```python
from build123d import *

# Parameters (mm, degrees)
SALIENTE_EXTRUIR1_DEPTH = 170
CROQUIS2_W              = 271.012090605
CROQUIS2_H              = 220
SALIENTE_EXTRUIR2_DEPTH = 2


with BuildPart() as part:
    # Croquis1 → Saliente-Extruir1 (new body)
    with BuildSketch(Plane(origin=(0, 0, 0), x_dir=(1, 0, 0), z_dir=(0, 1, 0))):
        Polygon((-305.737821636, -89.613714521), (-305.737821636, 100.579273879), (350.262178364, 100.579273879), (350.262178364, -117.420726121), (352.262178364, -117.420726121), (352.262178364, 102.579273879), (-307.737821636, 102.579273879), (-307.737821636, -89.613714521), align=None)
    extrude(amount=SALIENTE_EXTRUIR1_DEPTH)

    # Croquis2 → Saliente-Extruir2 (add)
    with BuildSketch(Plane(origin=(0, 170, 0), x_dir=(1, 0, 0), z_dir=(0, 1, 0))):
        with Locations((-172.231776334, -7.420726121)):
            Rectangle(CROQUIS2_W, CROQUIS2_H)
    extrude(amount=SALIENTE_EXTRUIR2_DEPTH)


solid = part.part
```
Here's how the part is built. I have some questions about the finished solid (model axes, mm). A direction names the side the tool comes from. Coordinates: 2 decimals unless noted, no trailing zeros. Loops run counter-clockwise (first coordinate to the right, second up) from the corner with the lowest first, then second, coordinate; pieces in that order, holes last. Notation, with made-up numbers: (15, 39) - (71, 39) arc R25 ccw to (71, 53) - close; hole circle Ø10 at (6, 12). An arc over 180 degrees is marked (long way). Answer as CSV lines item,"result".
Q1. If we section it at C-C, the plane x = -56: Write out the boundary of the cut face in (y, z), and give its area (3 significant figures).
Response:
outline,"(0, -102.58) - (172, -102.58) - (172, 117.42) - (170, 117.42) - (170, -100.58) - (0, -100.58) - close"
area,"780 mm2"
Q2. For faces 5 (the face through (350.262, 84, 7)), 6 (the face through (18, 85, -102.579)), 7 (the face through (18, 84, -100.579)), which set-ups out of +Z, -Z, +X, -X, +Y, -Y let a thin tool reach every point of the face, with its end or its side?
Response:
face 5,"+Z, +Y, -Y"
face 6,"-Z, +X, -X, +Y, -Y"
face 7,"+Z, -Y"
Q3. If we section it at D-D, the plane x = 278: Write out the boundary of the cut face in (y, z).
Response:
outline,"(0, -102.58) - (170, -102.58) - (170, -100.58) - (0, -100.58) - close"
Q4. If we section it at B-B, the plane y = 54: Write out the boundary of the cut face in (x, z).
Response:
outline,"(-307.74, -102.58) - (352.26, -102.58) - (352.26, 117.42) - (350.26, 117.42) - (350.26, -100.58) - (-305.74, -100.58) - (-305.74, 89.61) - (-307.74, 89.61) - close"
Q5. For pin 1 (3 mm diameter, centred on x = -134.5, z = 27.5, fed in from -Y); pin 2 (1.6 mm diameter, centred on x = -307, y = 125.5, fed in from +Z); pin 3 (0.6 mm diameter, centred on y = 171, z = 51.5, fed in from +X), each with a flat end and sliding along its axis, tell me the tip position at first contact or that it passes through.
Response:
pin 1,"y = 170"
pin 2,"z = 89.61"
pin 3,"x = -36.73"
Q6. If I drill on L1, parallel to X at y = 30.5, z = 53.5; L2, parallel to Z at x = 130, y = 28.5; L3, parallel to X at y = 45, z = 99.5, over which ranges is the centre line in solid material (lowest first)? Write a range as [from, to].
Response:
L1,"[-307.74, -305.74], [350.26, 352.26]"
L2,"[-102.58, -100.58]"
L3,"[350.26, 352.26]"
Q7. We'd pull the mould along X, two halves only. Please class faces 1 (the face through (352.262, 84, 9)), 2 (the face through (-305.738, 84, -4)), 3 (the face through (-174, 172, 6)), 4 (the face through (-307.738, 85, 9)): pulls with the +X half, pulls with the -X half, needs draft (parallel to the pull), parting line crosses it, or undercut.
Response:
face 1,"pulls with the +X half"
face 2,"undercut"
face 3,"needs draft"
face 4,"pulls with the -X half"
Q8. If we section it at A-A, the plane z = 64: Write out the boundary of the cut face in (x, y), and give its area (3 significant figures).
Response:
outline,"(-307.74, 0) - (-305.74, 0) - (-305.74, 170) - (-36.73, 170) - (-36.73, 172) - (-307.74, 172) - close; (350.26, 0) - (352.26, 0) - (352.26, 170) - (350.26, 170) - close"
area,"1,220 mm2"
